from build123d import *

# Parameters (mm, degrees)
F1_DEPTH = 0.28125


with BuildPart() as f1:
    # F0 (on Front) → F1 (new body)
    with BuildSketch(Plane.XZ):
        with BuildLine():
            ThreePointArc((-46.140093, -17.751075), (-44.007248, -36.292066), (-27.5, -45))
            Line((-27.5, -45), (27.5, -45))
            ThreePointArc((27.5, -45), (44.007248, -36.292066), (46.140093, -17.751075))
            Line((46.140093, -17.751075), (28.640093, 27.248925))
            ThreePointArc((28.640093, 27.248925), (21.292066, 36.507248), (10, 40))
            Line((10, 40), (0, 40))
            Line((0, 40), (-10, 40))
            ThreePointArc((-10, 40), (-21.292066, 36.507248), (-28.640093, 27.248925))
            Line((-28.640093, 27.248925), (-46.140093, -17.751075))
        make_face()
        with BuildLine():
            Line((-10, 30), (0, 30))
            Line((0, 30), (10, 30))
            ThreePointArc((10, 30), (15.646033, 28.253624), (19.320047, 23.624463))
            Line((19.320047, 23.624463), (36.820047, -21.375537))
            ThreePointArc((36.820047, -21.375537), (35.753624, -30.646033), (27.5, -35))
            Line((27.5, -35), (-27.5, -35))
            ThreePointArc((-27.5, -35), (-35.753624, -30.646033), (-36.820047, -21.375537))
            Line((-36.820047, -21.375537), (-19.320047, 23.624463))
            ThreePointArc((-19.320047, 23.624463), (-15.646033, 28.253624), (-10, 30))
        make_face(mode=Mode.SUBTRACT)
    extrude(amount=F1_DEPTH)


solid = f1.part
Source: CAD feature listing. Evaluate the final solid. Frame: model axes, mm. Coordinates: 2 decimals unless noted, no trailing zeros. Loops run counter-clockwise (first coordinate to the right, second up) from the corner with the lowest first, then second, coordinate; pieces in that order, holes last. Notation, with made-up numbers: (30, -17.5) - (45, -17.5) arc R22 cw to (45, 0.5) - close; hole circle Ø8 at (37.25, -19.75). An arc over 180 degrees is marked (long way). Return JSON: item names as keys, results as strings.
Q1. Section A-A, the plane y = -0.2. Return loops of the section in (x, z), plus the area to 3 significant figures.
Results:
{"outline": "(-46.14, -17.75) arc R20 ccw to (-27.5, -45) - (27.5, -45) arc R20 ccw to (46.14, -17.75) - (28.64, 27.25) arc R20 ccw to (10, 40) - (-10, 40) arc R20 ccw to (-28.64, 27.25) - close; hole (-36.82, -21.38) arc R10 ccw to (-27.5, -35) - (27.5, -35) arc R10 ccw to (36.82, -21.38) - (19.32, 23.62) arc R10 ccw to (10, 30) - (-10, 30) arc R10 ccw to (-19.32, 23.62) - close", "area": "2,660 mm2"}
Q2. Section C-C, the plane z = 0.5. Return loops of the section in (x, y).
Results:
{"outline": "(-39.04, -0.28) - (-28.31, -0.28) - (-28.31, 0) - (-39.04, 0) - close; (28.31, -0.28) - (39.04, -0.28) - (39.04, 0) - (28.31, 0) - close"}
Q3. Section B-B, the plane x = -20.5. Return loops of the section in (y, z), plus the area to 3 significant figures.
Results:
{"outline": "(-0.28, -45) - (0, -45) - (0, -35) - (-0.28, -35) - close; (-0.28, 20.59) - (0, 20.59) - (0, 37.02) - (-0.28, 37.02) - close", "area": "7.43 mm2"}
Q4. Material intervals for line 1 along Z through (x, y) = (9, -0.1); line 2 along X through (y, z) = (-0.05, 11.5); line 3 along X through (y, z) = (-0.15, 25.5), sorted ascending.
Results:
{"line 1": "-45 to -35, 30 to 40", "line 2": "-34.76 to -24.04, 24.04 to 34.76", "line 3": "-29.32 to -18.35, 18.35 to 29.32"}
